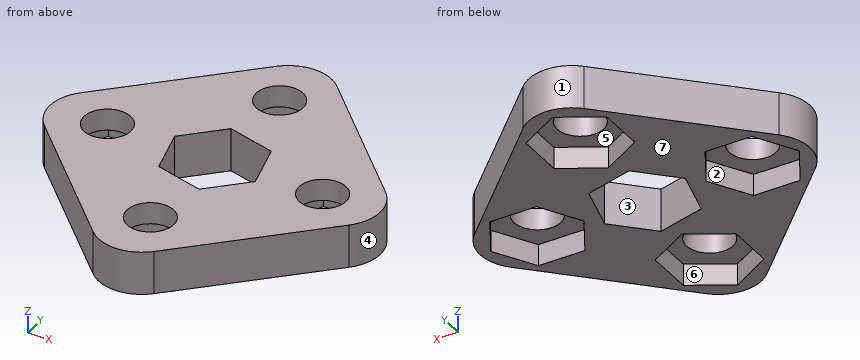
```python
from build123d import *

# Parameters (mm, degrees)
SKETCH2_R           = 3.429
BOSS_EXTRUDE1_DEPTH = 6.35
CUT_EXTRUDE1_DEPTH  = 3.175


with BuildPart() as part:
    # Sketch2 → Boss-Extrude1 (new body)
    with BuildSketch(Plane.XY):
        with BuildLine():
            Line((-4.490128061, 22.450640303), (-22.450640303, 4.490128061))
            ThreePointArc((-22.450640303, 4.490128061), (-24.310512242, 0), (-22.450640303, -4.490128061))
            Line((-22.450640303, -4.490128061), (-4.490128061, -22.450640303))
            ThreePointArc((-4.490128061, -22.450640303), (0, -24.310512242), (4.490128061, -22.450640303))
            Line((4.490128061, -22.450640303), (22.450640303, -4.490128061))
            ThreePointArc((22.450640303, -4.490128061), (24.310512242, 0), (22.450640303, 4.490128061))
            Line((22.450640303, 4.490128061), (4.490128061, 22.450640303))
            ThreePointArc((4.490128061, 22.450640303), (0, 24.310512242), (-4.490128061, 22.450640303))
        make_face()
        with Locations((0, 15.875)):
            Circle(SKETCH2_R, mode=Mode.SUBTRACT)
        with Locations((15.875, 0)):
            Circle(SKETCH2_R, mode=Mode.SUBTRACT)
        with Locations((0, -15.875)):
            Circle(SKETCH2_R, mode=Mode.SUBTRACT)
        with Locations((-15.875, 0)):
            Circle(SKETCH2_R, mode=Mode.SUBTRACT)
        Polygon((5.184753289, 5.184753289), (-1.897751416, 7.082504705), (-7.082504705, 1.897751416), (-5.184753289, -5.184753289), (1.897751416, -7.082504705), (7.082504705, -1.897751416), align=None, mode=Mode.SUBTRACT)
    extrude(amount=BOSS_EXTRUDE1_DEPTH)

    # Sketch3 → Cut-Extrude1 (cut)
    with BuildSketch(Plane(origin=(0, 0, 0), x_dir=(-1, 0, 0), z_dir=(0, 0, -1))):
        Polygon((5.953125, 19.312038321), (0, 22.749076643), (-5.953125, 19.312038321), (-5.953125, 12.437961679), (0, 9.000923357), (5.953125, 12.437961679), align=None)
        Polygon((12.437961679, -5.953125), (19.312038321, -5.953125), (22.749076643, 0), (19.312038321, 5.953125), (12.437961679, 5.953125), (9.000923357, 0), align=None)
        Polygon((-5.953125, -12.437961679), (-5.953125, -19.312038321), (0, -22.749076643), (5.953125, -19.312038321), (5.953125, -12.437961679), (0, -9.000923357), align=None)
        Polygon((-12.437961679, 5.953125), (-19.312038321, 5.953125), (-22.749076643, 0), (-19.312038321, -5.953125), (-12.437961679, -5.953125), (-9.000923357, 0), align=None)
    extrude(amount=-CUT_EXTRUDE1_DEPTH, mode=Mode.SUBTRACT)


solid = part.part
```
Build history of the part. All positions in model axes, mm. Face numbers are marked on the shaded views. A direction names the side the tool comes from. Give positions to 0.01 mm unless a question says otherwise; leave off trailing zeros. Loops run counter-clockwise (first coordinate to the right, second up) from the corner with the lowest first, then second, coordinate; pieces in that order, holes last. Notation, with made-up numbers: (38.25, -0.75) - (57.25, -0.75) arc R27 ccw to (57.25, 18.25) - close; hole circle Ø2 at (-24.75, -0.5). An arc over 180 degrees is marked (long way). Use a Markdown table: item, result.
(1) Pull direction X, two halves, no side cores. Call the marked faces 4, 5, 6 and 7: +X half, -X half, draft (parallel to the pull), parting line (faces both ways), or undercut.
Taken from the geometry:
| item | result |
|---|---|
| face 4 | +X half |
| face 5 | undercut |
| face 6 | undercut |
| face 7 | draft |
(2) Band-saw the part on C-C (z = 1.5). Give the number of separate pieces and of enclosed holes in the cut face, and give its area (3 significant figures).
Taken from the geometry:
| item | result |
|---|---|
| separate pieces | 1 |
| enclosed holes | 5 |
| area | 786 mm2 |
(3) Band-saw the part on A-A (y = -14). Give the cut face in (x, z) (3 decimals).
Taken from the geometry:
| item | result |
|---|---|
| outline | (-12.941, 0) - (-5.953, 0) - (-5.953, 3.175) - (-2.871, 3.175) - (-2.871, 6.35) - (-12.941, 6.35) - close; (2.871, 3.175) - (5.953, 3.175) - (5.953, 0) - (12.941, 0) - (12.941, 6.35) - (2.871, 6.35) - close |
(4) Drop flat-ended pins along their axis: pin 1 Ø6 at (x, y) = (-15, -2) entering from -Z (3 decimals); pin 2 Ø1 at (x, y) = (14, -14) entering from +Z; pin 3 Ø2 at (y, z) = (-2.5, 5.5) entering from +X; pin 4 Ø1 at (y, z) = (16.5, 1) entering from -X. Give the stop position or say it passes through.
Taken from the geometry:
| item | result |
|---|---|
| pin 1 | z = 3.175 |
| pin 2 | through |
| pin 3 | x = 24.13 |
| pin 4 | x = -10.94 |
(5) Wall check: line 1 along X through (y, z) = (0, 5.3); line 2 along X through (y, z) = (3, 2.5). Give the ranges that are in metal, low to high.
Taken from the geometry:
| item | result |
|---|---|
| line 1 | -24.31 to -19.3, -12.45 to -6.57, 6.57 to 12.45, 19.3 to 24.31 |
| line 2 | -23.56 to -21.02, -10.73 to -5.98, 5.77 to 10.73, 21.02 to 23.56 |
(6) Which spindle directions (+Z, -Z, +X, -X, +Y, -Y) get a long thin tool onto all of the face, cutting with end or side? Do the marked faces 1, 2 and 3. Say none if no direction does.
Taken from the geometry:
| item | result |
|---|---|
| face 1 | +Z, -Z, +Y |
| face 2 | -Z |
| face 3 | +Z, -Z |
(7) Band-saw the part on B-B (x = 1). Give the cut face in (y, z) (3 decimals).
Taken from the geometry:
| item | result |
|---|---|
| outline | (-24.231, 0) - (-22.172, 0) - (-22.172, 3.175) - (-19.155, 3.175) - (-19.155, 6.35) - (-24.231, 6.35) - close; (-12.595, 3.175) - (-9.578, 3.175) - (-9.578, 0) - (-6.842, 0) - (-6.842, 6.35) - (-12.595, 6.35) - close; (6.306, 0) - (9.578, 0) - (9.578, 3.175) - (12.595, 3.175) - (12.595, 6.35) - (6.306, 6.35) - close; (19.155, 3.175) - (22.172, 3.175) - (22.172, 0) - (24.231, 0) - (24.231, 6.35) - (19.155, 6.35) - close |
(8) Band-saw the part on D-D (y = 18.5). Give the cut face in (x, z) (3 decimals), and give its area (3 significant figures).
Taken from the geometry:
| item | result |
|---|---|
| outline | (-8.441, 0) - (-5.953, 0) - (-5.953, 3.175) - (-2.206, 3.175) - (-2.206, 6.35) - (-8.441, 6.35) - close; (2.206, 3.175) - (5.953, 3.175) - (5.953, 0) - (8.441, 0) - (8.441, 6.35) - (2.206, 6.35) - close |
| area | 55.4 mm2 |
